Autodesk Inventor part; units mm, degrees
ref_plane "YZ Plane" through (0, 0, 0) normal (1, 0, 0) x (0, 1, 0)
ref_plane "XZ Plane" through (0, 0, 0) normal (0, 1, 0) x (-1, 0, 0)
ref_plane "XY Plane" through (0, 0, 0) normal (0, 0, 1) x (1, 0, 0)
sketch "Sketch1" plane through (0, 0, 0) normal (0, 0, 1) x (1, 0, 0)
  line L0 (0, 0) -> (25.4, 0)
  line L1 (25.4, 0) -> (25.4, 25.4)
  line L2 (25.4, 25.4) -> (0, 25.4)
  line L3 (0, 25.4) -> (0, 0)
  line L4 (1.5875, 23.8125) -> (23.8125, 23.8125)
  line L5 (23.8125, 23.8125) -> (23.8125, 1.5875)
  line L6 (23.8125, 1.5875) -> (1.5875, 1.5875)
  line L7 (1.5875, 1.5875) -> (1.5875, 23.8125)
  dimension "d0" = 25.4
  dimension "d1" = 25.4
  dimension "d4" = 1.5875
extrude "Extrusion1" add sketch "Sketch1" against normal blind 25.4 contours L3 L2 L1 L0 | L4 L5 L6 L7
extrude "Extrusion2" add sketch "Sketch1" along normal blind 25.4 contours L4 L5 L6 L7
sketch "Sketch2" plane through (25.4, 0, 0) normal (1, 0, 0) x (0, 0, -1)
  line L0 (25.4, 0) -> (25.4, 25.4)
  line L1 (0, 25.4) -> (25.4, 25.4)
  line L2 (0, 0) -> (0, 25.4)
  line L3 (0, 0) -> (25.4, 0)
  line L4 (23.8125, 23.8125) -> (23.8125, 1.5875)
  line L5 (23.8125, 1.5875) -> (1.5875, 1.5875)
  line L6 (1.5875, 1.5875) -> (1.5875, 23.8125)
  line L7 (1.5875, 23.8125) -> (23.8125, 23.8125)
  dimension "d8" = 1.5875
sketch "Sketch3" plane through (0, 25.4, 0) normal (0, 1, 0) x (1, 0, 0)
  line L0 (25.4, 25.4) -> (0, 25.4)
  line L1 (0, 0) -> (0, 25.4)
  line L2 (25.4, 0) -> (0, 0)
  line L3 (25.4, 0) -> (25.4, 25.4)
  line L4 (1.5875, 23.8125) -> (23.8125, 23.8125)
  line L5 (23.8125, 23.8125) -> (23.8125, 1.5875)
  line L6 (23.8125, 1.5875) -> (1.5875, 1.5875)
  line L7 (1.5875, 1.5875) -> (1.5875, 23.8125)
  dimension "d9" = 1.5875
extrude "Extrusion3" add sketch "Sketch2" along normal blind 25.4 contours L4 L5 L6 L7
extrude "Extrusion4" add sketch "Sketch3" along normal blind 25.4 contours L4 L5 L6 L7
sketch "Sketch4" plane through (0, 0, 0) normal (-1, 0, 0) x (0, 0, 1)
  line L0 (-25.4, 25.4) -> (-25.4, 0)
  line L1 (0, 0) -> (-25.4, 0)
  line L2 (0, 25.4) -> (0, 0)
  line L3 (0, 25.4) -> (-25.4, 25.4)
  line L4 (-23.8125, 23.8125) -> (-23.8125, 1.5875)
  line L5 (-23.8125, 1.5875) -> (-1.5875, 1.5875)
  line L6 (-1.5875, 1.5875) -> (-1.5875, 23.8125)
  line L7 (-1.5875, 23.8125) -> (-23.8125, 23.8125)
  dimension "d15" = 1.5875
extrude "Extrusion5" add sketch "Sketch4" along normal blind 25.4 contours L7 L6 L5 L4
sketch "Sketch6" plane through (0, 23.8125, -1.5875) normal (0, 1, 0) x (1, 0, 0)
  line L0 (-25.4, 22.225) -> (-25.4, 0)
  line L1 (0, 22.225) -> (0, 0)
  line L2 (0, 22.225) -> (-25.4, 22.225)
  line L3 (25.4, -1.5875) -> (0, -1.5875)
  point P0 (-12.7, 11.1125)
  point P1 (12.7, -14.2875)
  point P2 (38.1, 11.1125)
  dimension "d21" = 12.7
  dimension "d22" = 50.8
  dimension "d23" = 11.1125
  dimension "d24" = 12.7
  dimension "d25" = 12.7
hole "Hole1" at (-12.7, 23.8125, -12.7) at (12.7, 23.8125, 12.7) at (38.1, 23.8125, -12.7) direction (0, -1, 0) diameter 6.35 depth 25.4 tip angle 118
sketch "Sketch7" plane through (23.8125, 25.4, -23.8125) normal (0, 0, -1) x (-1, 0, 0)
  point P0 (23.8125, -25.4)
  point P1 (11.1125, 12.7)
hole "Hole2" at (12.7, 38.1, -23.8125) direction (0, 0, 1) diameter 6.35 depth 25.4 tip angle 118
sketch "Sketch8" plane through (1.5875, 25.4, -23.8125) normal (-1, 0, 0) x (0, 0, 1)
  point P0 (23.8125, -25.4)
  point P1 (11.1125, 12.7)
hole "Hole3" at (1.5875, 38.1, -12.7) direction (1, 0, 0) diameter 6.35 depth 25.4 tip angle 118
properties part number "4-way corner"
Source: CAD feature listing. Evaluate the final solid. Frame: model axes, mm. A direction names the side the tool comes from. Give positions to 0.01 mm unless a question says otherwise; leave off trailing zeros. Write each loop counter-clockwise with the first axis right and the second up, starting at its lowest first coordinate (ties: lowest second). Pieces come first, ordered by that corner, then holes. Notation, with made-up numbers: M 85,39 L 108,39 A13 ccw 108,61 Z; hole C 10.5,66 d7. An arc over 180 degrees is marked long. Answer as a JSON object with one key per item and string values.
Q1. Access query for faces 4 (the face through (1.588, 13, 13)), 5 (the face through (10, 23.812, 15)), 6 (the face through (23.812, 35, -15)). Directions: +Z, -Z, +X, -X, +Y, -Y. A direction counts if a zero-diameter tool reaches every point of the face in a straight line with its end or side. Return the directions, or none.
Geometry check:
{"face 4": "+Z, -X, +Y, -Y", "face 5": "+Z, +X, -X, +Y", "face 6": "+Z, -Z, +X, +Y"}
Q2. Cut plane B-B, the plane x = -12.7. Return the cut outline in (y, z) (1 decimal).
Geometry check:
{"outline": "M 1.6,-23.8 L 23.8,-23.8 L 23.8,-15.9 L 1.6,-15.9 Z; M 1.6,-9.5 L 23.8,-9.5 L 23.8,-1.6 L 1.6,-1.6 Z"}
Q3. Cut plane A-A, the plane z = 12.7. Return the cut outline in (x, y) (1 decimal).
Geometry check:
{"outline": "M 1.6,1.6 L 9.5,1.6 L 9.5,23.8 L 1.6,23.8 Z; M 15.9,1.6 L 23.8,1.6 L 23.8,23.8 L 15.9,23.8 Z"}
Q4. Ray query, line 1 along Y through (x, z) = (19, -12.7) (3 decimals); line 2 along Y through (x, z) = (0.5, -9); line 3 along Z through (x, y) = (21, 38). Return the intervals inside material, ascending.
Geometry check:
{"line 1": "y = 0 to 34.925, 41.275 to 50.8", "line 2": "y = 0 to 25.4", "line 3": "z = -23.81 to -15.87, -9.53 to -1.59"}
Q5. Cut plane C-C, the plane y = 38.1. Return the cut outline in (x, z) (1 decimal).
Geometry check:
{"outline": "M 1.6,-23.8 L 9.5,-23.8 L 9.5,-15.9 L 1.6,-15.9 Z; M 1.6,-9.5 L 9.5,-9.5 L 9.5,-1.6 L 1.6,-1.6 Z; M 15.9,-23.8 L 23.8,-23.8 L 23.8,-15.9 L 15.9,-15.9 Z; M 15.9,-9.5 L 23.8,-9.5 L 23.8,-1.6 L 15.9,-1.6 Z"}
Q6. Mould query, pull axis Z, two halves, no side actions, for faces 1 (the face through (38, 13, -1.588)), 2 (the face through (15.3, 1.588, 15.3)), 3 (the face through (19.57, 37.15, -9.67)). Classes: +Z half, -Z half, draft (parallel to the pull), parting line (faces both ways), or undercut.
Geometry check:
{"face 1": "+Z half", "face 2": "draft", "face 3": "undercut"}
Q7. Contact query for flat-ended pins moving along their axis: P1, Ø11, axis at x = 8.5, y = 34, coming from the +Z side; P2, Ø10, axis at y = 38.1, z = -12.7, coming from the -X side; P3, Ø11, axis at x = -18.5, z = -9.5, coming from the -Y side; P4, Ø3, axis at x = -1, z = 6, coming from the +Y side. Output: stop coordinate, or through.
Geometry check:
{"P1": "stops at z = -1.59", "P2": "stops at x = 1.59", "P3": "stops at y = 1.59", "P4": "passes through"}
